from build123d import *

# Parameters (mm, degrees)
F0_W     = 165.1
F0_H     = 19.05
F1_DEPTH = 3.175
F2_R     = 1.4986
F3_DEPTH = 25.4
F2_R_2   = 0.9779
F4_DEPTH = 25.4
F5_DEPTH = 25.4
F2_W     = 22.225
F2_H     = 11.938
F6_DEPTH = 22.225


with BuildPart() as f1:
    # F0 (on Top) → F1 (new body)
    with BuildSketch(Plane.XY):
        with Locations((-49.068541, -18.8957)):
            Rectangle(F0_W, F0_H)
    extrude(amount=F1_DEPTH)

    # F2 (on face) → F3 (cut)
    with BuildSketch(Plane(origin=(0, 0, 0), x_dir=(1, 0, 0), z_dir=(0, 0, -1))):
        with Locations((-39.137141, 18.8957)):
            Circle(F2_R)
    extrude(amount=-F3_DEPTH, mode=Mode.SUBTRACT)

    # F2 (on face) → F4 (cut)
    with BuildSketch(Plane(origin=(0, 0, 0), x_dir=(1, 0, 0), z_dir=(0, 0, -1))):
        with Locations((-60.137141, 18.8957)):
            Circle(F2_R_2)
    extrude(amount=-F4_DEPTH, mode=Mode.SUBTRACT)

    # F2 (on face) → F5 (cut)
    with BuildSketch(Plane(origin=(0, 0, 0), x_dir=(1, 0, 0), z_dir=(0, 0, -1))):
        with Locations((-9.143541, 18.8957)):
            Circle(F2_R)
    extrude(amount=-F5_DEPTH, mode=Mode.SUBTRACT)

    # F2 (on face) → F6 (join)
    with BuildSketch(Plane(origin=(0, 0, 0), x_dir=(1, 0, 0), z_dir=(0, 0, -1))):
        with Locations((-3.031041, 18.8957)):
            Rectangle(F2_W, F2_H)
        with Locations((-9.143541, 18.8957)):
            Circle(F2_R, mode=Mode.SUBTRACT)
    extrude(amount=F6_DEPTH)


solid = f1.part
CAD build for the part. Positions are in the model's coordinates, mm. A direction names the side the tool comes from. Round coordinates to 2 decimals unless told otherwise and drop trailing zeros. Write each loop counter-clockwise with the first axis right and the second up, starting at its lowest first coordinate (ties: lowest second). Pieces come first, ordered by that corner, then holes. Notation, with made-up numbers: M 86,79.5 L 138,79.5 A23 ccw 138,112.5 Z; hole C -32,-25 d5. An arc over 180 degrees is marked long. Use a Markdown table: item, result. Add a question column.
1. 3-axis set-ups, long thin cutter, end or side, ignore diameter. For faces 1 (the face through (-3, -24.865, -11)), 2 (the face through (8.081, -19, -11)), 3 (the face through (-14.144, -19, -11)): which of +Z, -Z, +X, -X, +Y, -Y reach the whole face in a straight line?
2. Slice it at D-D on x = -79.5. Give the cut face in (y, z) (3 decimals).
3. Slice it at C-C on y = -11.5. Give the cut face in (x, z) (3 decimals), then the cut area to 3 significant figures.
4. Flat gauge pins, fed straight in: P1, Ø6.5, axis at x = -3.5, z = -8, coming from the +Y side; P2, Ø8, axis at y = -22.5, z = -18, coming from the -X side; P3, Ø2.5, axis at x = -9.14, y = -18.9, coming from the +Z side; P4, Ø4, axis at x = -39.14, y = -18.9, coming from the -Z side. Where does each tip first touch, or does it go through?
5. Slice it at A-A on x = 4. Give the cut face in (y, z) (3 decimals), then the cut area to 3 significant figures.
6. Drill centre lines: probe 1 along Z at (x, y) = (-59.5, -21.75) (3 decimals); probe 2 along X at (y, z) = (-15.5, -9.5); probe 3 along Y at (x, z) = (3, -10.5). Where is each one in solid material? Low to high.
7. Slice it at B-B on z = -8. Give the cut face in (x, y), then the cut area to 3 significant figures.
Reply:
| question | item | result |
|---|---|---|
| 1 | face 1 | -Z, +X, -X, -Y |
| 1 | face 2 | -Z, +X, +Y, -Y |
| 1 | face 3 | -Z, -X, +Y, -Y |
| 2 | outline | M -28.421,0 L -9.371,0 L -9.371,3.175 L -28.421,3.175 Z |
| 3 | outline | M -131.619,0 L 33.481,0 L 33.481,3.175 L -131.619,3.175 Z |
| 3 | area | 524 mm^2 |
| 4 | P1 | stops at y = -12.93 |
| 4 | P2 | stops at x = -14.14 |
| 4 | P3 | passes through |
| 4 | P4 | stops at z = 0 |
| 5 | outline | M -28.421,0 L -24.865,0 L -24.865,-22.225 L -12.927,-22.225 L -12.927,0 L -9.371,0 L -9.371,3.175 L -28.421,3.175 Z |
| 5 | area | 326 mm^2 |
| 6 | probe 1 | z = 0 to 3.175 |
| 6 | probe 2 | x = -14.14 to 8.08 |
| 6 | probe 3 | y = -24.86 to -12.93 |
| 7 | outline | M -14.14,-24.86 L 8.08,-24.86 L 8.08,-12.93 L -14.14,-12.93 Z; hole C -9.14,-18.9 d3 |
| 7 | area | 258 mm^2 |
